Input: part model. Units: mm. Frame: model coordinates. Face numbers are marked on the shaded views. Give positions to 0.01 mm unless a question says otherwise; leave off trailing zeros. Loops run counter-clockwise (first coordinate to the right, second up) from the corner with the lowest first, then second, coordinate; pieces in that order, holes last. Notation, with made-up numbers: (17, 10.25) - (63, 10.25) arc R24 ccw to (63, 23.25) - close; hole circle Ø3 at (7, -37.5). An arc over 180 degrees is marked (long way). Answer as a JSON object with one key per item and string values.
from build123d import *

# Parameters (mm, degrees)
SKETCH1_R           = 9.5
SKETCH1_R_2         = 2
BOSS_EXTRUDE1_DEPTH = 20
SKETCH3_R           = 5
CUT_EXTRUDE1_DEPTH  = 10


with BuildPart() as part:
    # Sketch1 → Boss-Extrude1 (new body)
    with BuildSketch(Plane(origin=(0, 0, 0), x_dir=(1, 0, 0), z_dir=(0, 1, 0))):
        with Locations(Location((0, 0, 0), (0, 0, 270))):
            Circle(SKETCH1_R)
        with Locations(Location((0, 0, 0), (0, 0, 270))):
            Circle(SKETCH1_R_2, mode=Mode.SUBTRACT)
    extrude(amount=BOSS_EXTRUDE1_DEPTH)

    # Sketch2 → Cut-Revolve1 (revolve, cut)
    with BuildSketch(Plane.XY, mode=Mode.PRIVATE) as cut_revolve1_sk:
        Polygon((-9.5, 20), (-8.5, 0), (-9.5, 0), align=None)
    revolve(cut_revolve1_sk.sketch.rotate(Axis((0, 20, 0), (0, -1, 0)), 270), axis=Axis((0, 20, 0), (0, -1, 0)), mode=Mode.SUBTRACT)

    # Sketch3 → Cut-Extrude1 (cut)
    with BuildSketch(Plane.XZ):
        with Locations(Location((0, 0, 0), (0, 0, 270))):
            Circle(SKETCH3_R)
    extrude(amount=-CUT_EXTRUDE1_DEPTH, mode=Mode.SUBTRACT)


solid = part.part
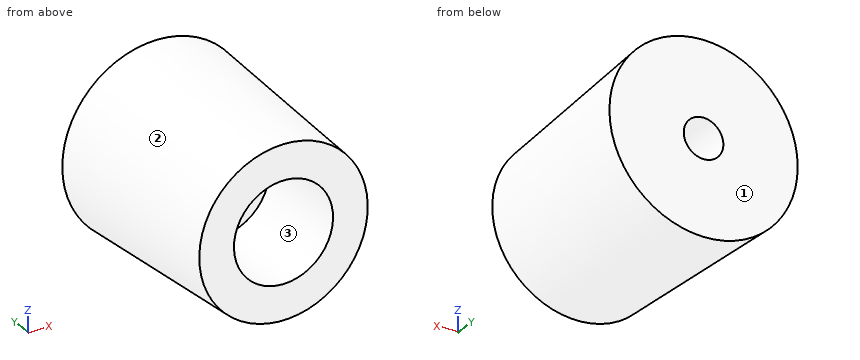
Item 1: Material intervals for line 1 (X direction, y = 3.5, z = 0) (3 decimals); line 2 (Y direction, x = 3.75, z = -2.5); line 3 (X direction, y = 15.5, z = 0) (3 decimals), sorted ascending. Write a range as [from, to].
Geometry check:
{"line 1": "x = [-8.675, -5], [5, 8.675]", "line 2": "y = [10, 20]", "line 3": "x = [-9.275, -2], [2, 9.275]"}
Item 2: Cut plane B-B (z = 0). Return loops of the section in (x, y), then the cut area to 3 significant figures.
Geometry check:
{"outline": "(-9.5, 20) - (-8.5, 0) - (-5, 0) - (-5, 10) - (-2, 10) - (-2, 20) - close; (2, 10) - (5, 10) - (5, 0) - (8.5, 0) - (9.5, 20) - (2, 20) - close", "area": "220 mm2"}
Item 3: Cut plane C-C (y = 7). Return loops of the section in (x, z), then the cut area to 3 significant figures.
Geometry check:
{"outline": "circle Ø17.7 at (0, 0); hole circle Ø10 at (0, 0)", "area": "168 mm2"}
Item 4: Contact query for flat-ended pins moving along their axis: P1, Ø2.5, axis at x = 0, z = 0, coming from the +Y side; P2, Ø9, axis at x = 0, z = 0, coming from the -Y side; P3, Ø4, axis at x = 7, y = 5.5, coming from the -Z side; P4, Ø1.5, axis at x = -7.5, y = 9, coming from the -Z side. Output: stop coordinate, or through.
Geometry check:
{"P1": "passes through", "P2": "stops at y = 10", "P3": "stops at z = -7.22", "P4": "stops at z = -5.88"}
Item 5: Cut plane D-D (y = 14.5). Return loops of the section in (x, z) (3 decimals).
Geometry check:
{"outline": "circle Ø18.45 at (0, 0); hole circle Ø4 at (0, 0)"}
Item 6: Cut plane A-A (x = 0). Return loops of the section in (y, z).
Geometry check:
{"outline": "(0, -8.5) - (20, -9.5) - (20, -2) - (10, -2) - (10, -5) - (0, -5) - close; (0, 5) - (10, 5) - (10, 2) - (20, 2) - (20, 9.5) - (0, 8.5) - close"}
Item 7: Mould query, pull axis Z, two halves, no side actions, for the marked faces 1, 2 and 3. Classes: released by +Z, released by -Z, zero draft, split by the parting line, or undercut.
Geometry check:
{"face 1": "zero draft", "face 2": "split by the parting line", "face 3": "undercut"}
